Geometry check sheet. Reference: drawing and pictorial views, mm from the part's lowest x, y, z. A direction names the side the tool comes from. Coordinates: 2 decimals unless noted, no trailing zeros. Loops run counter-clockwise (first coordinate to the right, second up) from the corner with the lowest first, then second, coordinate; pieces in that order, holes last. Notation, with made-up numbers: (74, -36) -> (80, -36) arc R16 ccw to (80, -19) -> close; hole circle Ø3 at (75.5, -22). An arc over 180 degrees is marked (long way). Use CSV: the item, a comma, the result in double quotes.
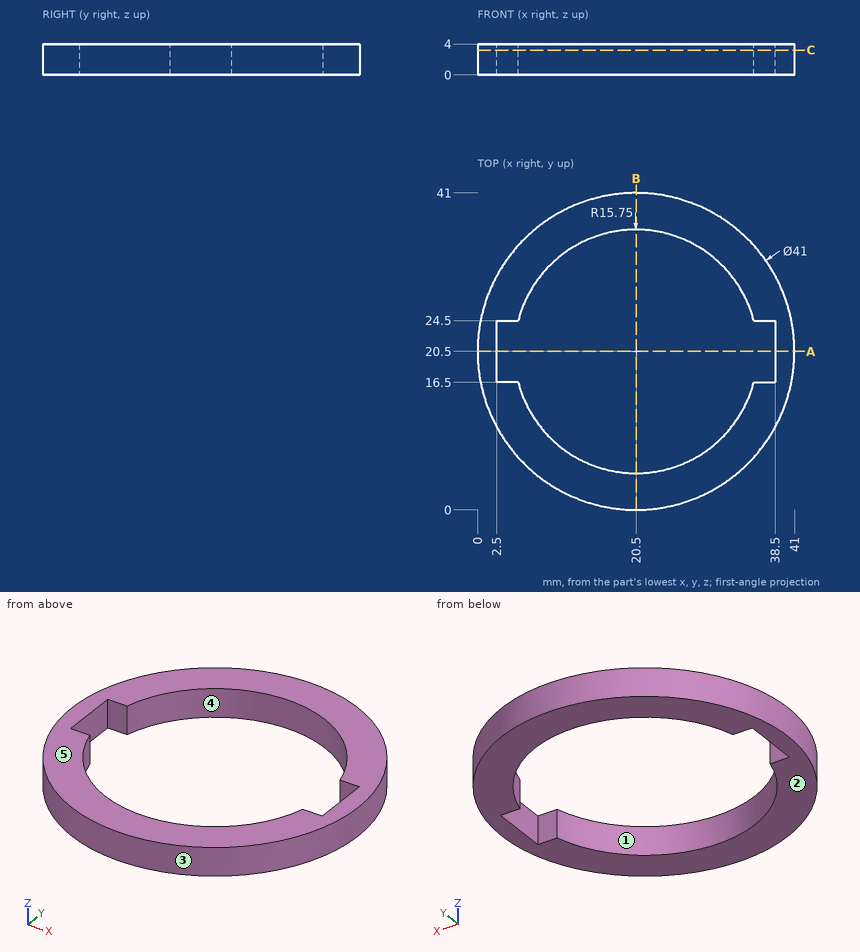
1) Cross-section at A-A on y = 20.5. Record the boundary of the cut face in (x, z), and give its area (3 significant figures).
Answer below:
outline,"(0, 0) -> (2.5, 0) -> (2.5, 4) -> (0, 4) -> close; (38.5, 0) -> (41, 0) -> (41, 4) -> (38.5, 4) -> close"
area,"20.0 mm²"
2) Access from +Z, -Z, +X, -X, +Y, -Y to the whole of each face (thin tool, end or side, straight path). Record for the marked faces 4 and 5.
Answer below:
face 4,"+Z, -Z"
face 5,"+Z, +X, -X, +Y, -Y"
3) Draft check along X on the marked faces 1, 2 and 3. Enter one of: released by +X, released by -X, zero draft, split by the parting line, or undercut.
Answer below:
face 1,"undercut"
face 2,"zero draft"
face 3,"split by the parting line"
4) Go/stop test with flat-tipped pins: pin 1 Ø1.2 at (y, z) = (19.5, 1.5) entering from -X; pin 2 Ø2 at (x, z) = (37, 2.5) entering from +Y; pin 3 Ø2 at (x, z) = (4, 1.5) entering from -Y. Record where each tip stops, or that it passes through.
Answer below:
pin 1,"stops at x = 0"
pin 2,"stops at y = 33.92"
pin 3,"stops at y = 7.08"
5) Cross-section at B-B on x = 20.5. Record the boundary of the cut face in (y, z), and give its area (3 significant figures).
Answer below:
outline,"(0, 0) -> (4.75, 0) -> (4.75, 4) -> (0, 4) -> close; (36.25, 0) -> (41, 0) -> (41, 4) -> (36.25, 4) -> close"
area,"38.0 mm²"
6) Cross-section at C-C on z = 3.2. Record the boundary of the cut face in (x, y), and give its area (3 significant figures).
Answer below:
outline,"circle Ø41 at (20.5, 20.5); hole (2.5, 16.5) -> (5.27, 16.5) arc R15.75 ccw to (35.73, 16.5) -> (38.5, 16.5) -> (38.5, 24.5) -> (35.73, 24.5) arc R15.75 ccw to (5.27, 24.5) -> (2.5, 24.5) -> close"
area,"502 mm²"
7) Thickness scan on line 1 along Y through (x, z) = (21, 2.7); line 2 along X through (y, z) = (19.5, 3); line 3 along Y through (x, z) = (32, 1). Record the ranges inside material, lowest first. Write a range as from..to.
Answer below:
line 1,"y = 0.01..4.76, 36.24..40.99"
line 2,"x = 0.02..2.5, 38.5..40.98"
line 3,"y = 3.53..9.74, 31.26..37.47"
